Print and shaded views of the part. All mm, measured from the part's lowest x, y and z. Give positions to 0.01 mm unless a question says otherwise; leave off trailing zeros. Write each loop counter-clockwise with the first axis right and the second up, starting at its lowest first coordinate (ties: lowest second). Pieces come first, ordered by that corner, then holes. Notation, with made-up numbers: M 47.25,-3 L 69.25,-3 A10 ccw 69.25,15 Z; hole C 49,-3 d9. An arc over 180 degrees is marked long. One line per question, with ' | ' between items. Start each with the question number.
1. Flat gauge pins, fed straight in: pin 1 (10 mm diameter, centred on x = 24, z = 28, fed in from -Y); pin 2 (1.5 mm diameter, centred on x = 36, z = 4, fed in from +Y); pin 3 (4.5 mm diameter, centred on x = 65.09, z = 19.05, fed in from -Y); pin 4 (6.5 mm diameter, centred on x = 14.29, z = 19.05, fed in from +Y). Where does each tip first touch, or does it go through?
2. Wall check: L1, parallel to X at y = 17.25, z = 19.05 (1 decimal); L2, parallel to Y at x = 59.5, z = 8; L3, parallel to Y at x = 60.5, z = 33. Give the ranges that are in metal, low to high.
3. Cut at A-A, the plane x = 32. Write the cut outline in (y, z).
4. Cut at B-B, the plane z = 33.5. Write the cut outline in (x, y) (1 decimal), then the cut area to 3 significant figures.
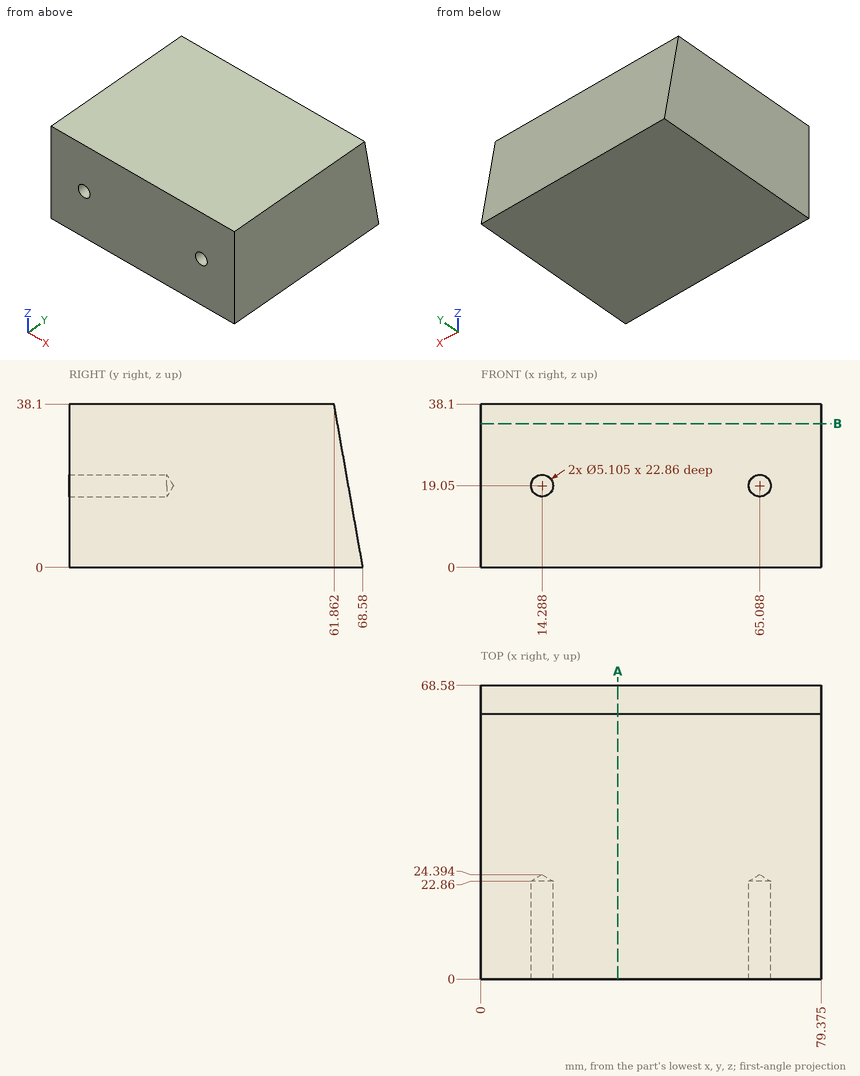
Here are the results:
1) pin 1: y = 0 | pin 2: y = 68.01 | pin 3: y = 23.04 | pin 4: y = 65.79
2) L1: 0 to 11.7, 16.8 to 62.5, 67.6 to 79.4 | L2: 0 to 67.17 | L3: 0 to 62.76
3) outline: M 0,0 L 68.58,0 L 61.86,38.1 L 0,38.1 Z
4) outline: M 0,0 L 79.4,0 L 79.4,62.7 L 0,62.7 Z | area: 4,970 mm^2
